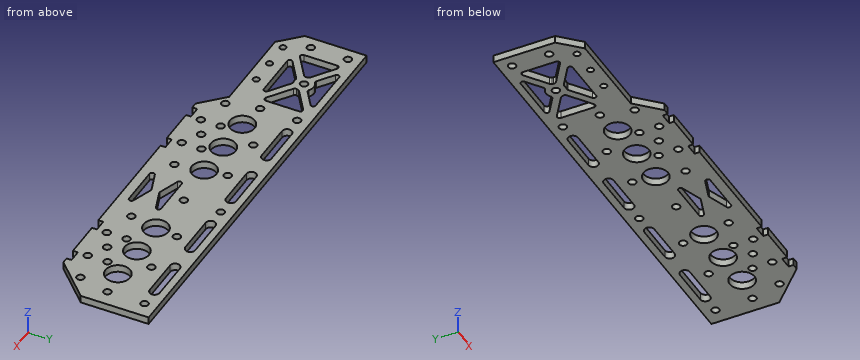
from build123d import *

# Parameters (mm, degrees)
SKETCH_1_R          = 1.55
SKETCH_1_R_2        = 1.3
EXTRUDE_1_DEPTH     = 3
FILLET_1_R          = 1
SKETCH_2_R          = 5
SKETCH_2_R_2        = 1.55
CUT_EXTRUDE_1_DEPTH = 10
SKETCH_3_W          = 5
SKETCH_3_H          = 8
CUT_EXTRUDE_2_DEPTH = 10


with BuildPart() as part:
    # 草图1 → 凸台-拉伸1 (new body)
    with BuildSketch(Plane.XY):
        Polygon((-68, 32), (103.45, 32), (103.45, 7), (103.45, 4.5), (88.907352941, -10), (86.4, -10), (-12.5, -10), (-15, -10), (-24.026470588, -1), (-60.023460411, -1), (-68, 7), align=None)
        with Locations((-7.5, 4)):
            Circle(SKETCH_1_R, mode=Mode.SUBTRACT)
        with Locations((-7.5, -4)):
            Circle(SKETCH_1_R, mode=Mode.SUBTRACT)
        with Locations((7.5, -4)):
            Circle(SKETCH_1_R, mode=Mode.SUBTRACT)
        with Locations((7.5, 4)):
            Circle(SKETCH_1_R, mode=Mode.SUBTRACT)
        with Locations((66.4, 4)):
            Circle(SKETCH_1_R, mode=Mode.SUBTRACT)
        with Locations((66.4, -4)):
            Circle(SKETCH_1_R, mode=Mode.SUBTRACT)
        with Locations((81.4, 4)):
            Circle(SKETCH_1_R, mode=Mode.SUBTRACT)
        with Locations((81.4, -4)):
            Circle(SKETCH_1_R, mode=Mode.SUBTRACT)
        with Locations((-63, 27)):
            Circle(SKETCH_1_R, mode=Mode.SUBTRACT)
        with Locations((-63, 12)):
            Circle(SKETCH_1_R, mode=Mode.SUBTRACT)
        with Locations((16.95, 19.5)):
            Circle(SKETCH_1_R, mode=Mode.SUBTRACT)
        with Locations((-3.05, 19.5)):
            Circle(SKETCH_1_R, mode=Mode.SUBTRACT)
        with Locations((-23.05, 27)):
            Circle(SKETCH_1_R, mode=Mode.SUBTRACT)
        with Locations((-23.05, 12)):
            Circle(SKETCH_1_R, mode=Mode.SUBTRACT)
        with Locations((36.95, 27)):
            Circle(SKETCH_1_R, mode=Mode.SUBTRACT)
        with Locations((36.95, 12)):
            Circle(SKETCH_1_R, mode=Mode.SUBTRACT)
        with Locations((56.95, 19.5)):
            Circle(SKETCH_1_R, mode=Mode.SUBTRACT)
        with Locations((76.95, 19.5)):
            Circle(SKETCH_1_R, mode=Mode.SUBTRACT)
        with Locations((96.95, 27)):
            Circle(SKETCH_1_R, mode=Mode.SUBTRACT)
        with Locations((96.95, 12)):
            Circle(SKETCH_1_R, mode=Mode.SUBTRACT)
        with Locations((-48, 3)):
            Circle(SKETCH_1_R_2, mode=Mode.SUBTRACT)
        with Locations((-37.5, 3)):
            Circle(SKETCH_1_R_2, mode=Mode.SUBTRACT)
        with Locations((-58.5, 3)):
            Circle(SKETCH_1_R_2, mode=Mode.SUBTRACT)
        with Locations((-43.05, 19.5)):
            Circle(SKETCH_1_R, mode=Mode.SUBTRACT)
        with Locations((93.9, -0.5)):
            Circle(SKETCH_1_R, mode=Mode.SUBTRACT)
        with Locations(Location((53.9, -0.5, 0), (0, 0, 180))):
            Circle(SKETCH_1_R, mode=Mode.SUBTRACT)
        with Locations(Location((-20, -0.5, 0), (0, 0, 180))):
            Circle(SKETCH_1_R, mode=Mode.SUBTRACT)
        with Locations((20, -0.5)):
            Circle(SKETCH_1_R, mode=Mode.SUBTRACT)
        with BuildLine():
            Line((-15.05, 29), (0.95, 29))
            ThreePointArc((0.95, 29), (2.95, 27), (0.95, 25))
            Line((0.95, 25), (-15.05, 25))
            ThreePointArc((-15.05, 25), (-17.05, 27), (-15.05, 29))
        make_face(mode=Mode.SUBTRACT)
        with BuildLine():
            Line((12.95, 29), (28.95, 29))
            ThreePointArc((28.95, 29), (30.95, 27), (28.95, 25))
            Line((28.95, 25), (12.95, 25))
            ThreePointArc((12.95, 25), (10.95, 27), (12.95, 29))
        make_face(mode=Mode.SUBTRACT)
        with BuildLine():
            Line((44.95, 29), (60.95, 29))
            ThreePointArc((60.95, 29), (62.95, 27), (60.95, 25))
            Line((60.95, 25), (44.95, 25))
            ThreePointArc((44.95, 25), (42.95, 27), (44.95, 29))
        make_face(mode=Mode.SUBTRACT)
        with BuildLine():
            Line((72.95, 29), (88.95, 29))
            ThreePointArc((88.95, 29), (90.95, 27), (88.95, 25))
            Line((88.95, 25), (72.95, 25))
            ThreePointArc((72.95, 25), (70.95, 27), (72.95, 29))
        make_face(mode=Mode.SUBTRACT)
        with BuildLine():
            Line((-30.662765464, 29), (-40.203557385, 22.310296148))
            ThreePointArc((-40.203557385, 22.310296148), (-43.03543461, 23.499973481), (-45.875900736, 22.330951259))
            Line((-45.875900736, 22.330951259), (-55.387234536, 29))
            Line((-55.387234536, 29), (-30.662765464, 29))
        make_face(mode=Mode.SUBTRACT)
        with BuildLine():
            Line((-55.387234536, 8), (-44.370821033, 15.724363392))
            ThreePointArc((-44.370821033, 15.724363392), (-43.032385745, 15.500038783), (-41.695978002, 15.736142347))
            Line((-41.695978002, 15.736142347), (-30.662765464, 8))
            Line((-30.662765464, 8), (-55.387234536, 8))
        make_face(mode=Mode.SUBTRACT)
        with BuildLine():
            Line((-58, 27.16801086), (-47.04998801, 19.490206126))
            ThreePointArc((-47.04998801, 19.490206126), (-46.950749965, 18.614477719), (-46.662143081, 17.781738565))
            Line((-46.662143081, 17.781738565), (-58, 9.83198914))
            Line((-58, 9.83198914), (-58, 27.16801086))
        make_face(mode=Mode.SUBTRACT)
        with BuildLine():
            Line((-39.425439217, 17.808090093), (-28.05, 9.83198914))
            Line((-28.05, 9.83198914), (-28.05, 27.16801086))
            Line((-28.05, 27.16801086), (-39.050253376, 19.454978443))
            ThreePointArc((-39.050253376, 19.454978443), (-39.149926133, 18.611504738), (-39.425439217, 17.808090093))
        make_face(mode=Mode.SUBTRACT)
        Polygon((23.014193592, -6), (36.95, -1.090366306), (50.885806408, -6), align=None, mode=Mode.SUBTRACT)
        Polygon((23.014193592, 7), (36.95, 2.090366306), (50.885806408, 7), align=None, mode=Mode.SUBTRACT)
    extrude(amount=EXTRUDE_1_DEPTH)

    # 圆角1
    fillet_1_edges = [part.edges().sort_by_distance(p)[0] for p in [
        (-30.662765464, 29, 1.5),
        (-55.387234536, 29, 1.5),
        (-45.875900736, 22.330951259, 1.5),
        (-40.203557385, 22.310296148, 1.5),
        (-55.387234536, 8, 1.5),
        (-30.662765464, 8, 1.5),
        (-41.695978002, 15.736142347, 1.5),
        (-44.370821033, 15.724363392, 1.5),
        (-58, 27.16801086, 1.5),
        (-58, 9.83198914, 1.5),
        (-46.662143081, 17.781738565, 1.5),
        (-47.04998801, 19.490206126, 1.5),
        (-28.05, 9.83198914, 1.5),
        (-28.05, 27.16801086, 1.5),
        (-39.050253376, 19.454978443, 1.5),
        (-39.425439217, 17.808090093, 1.5),
        (50.885806408, 7, 1.5),
        (23.014193592, 7, 1.5),
        (36.95, 2.090366306, 1.5),
        (23.014193592, -6, 1.5),
        (50.885806408, -6, 1.5),
        (36.95, -1.090366306, 1.5),
    ]]
    fillet(fillet_1_edges, radius=FILLET_1_R)

    # 草图2 → 切除-拉伸1 (cut)
    with BuildSketch(Plane.XY.offset(3)):
        with Locations((-12, 10.5)):
            Circle(SKETCH_2_R)
        with Locations((3, 10.5)):
            Circle(SKETCH_2_R)
        with Locations((18, 10.5)):
            Circle(SKETCH_2_R)
        with Locations(Location((55.907352941, 10.5, 0), (0, 0, 180))):
            Circle(SKETCH_2_R)
        with Locations(Location((70.907352941, 10.5, 0), (0, 0, 180))):
            Circle(SKETCH_2_R)
        with Locations(Location((85.907352941, 10.5, 0), (0, 0, 180))):
            Circle(SKETCH_2_R)
        Circle(SKETCH_2_R_2)
        with Locations(Location((73.907352941, 0, 0), (0, 0, 180))):
            Circle(SKETCH_2_R_2)
    extrude(amount=-CUT_EXTRUDE_1_DEPTH, mode=Mode.SUBTRACT)

    # 草图3 → 切除-拉伸2 (cut)
    with BuildSketch(Plane.XY.offset(3)):
        with Locations((-10, -12)):
            Rectangle(SKETCH_3_W, SKETCH_3_H)
        with Locations((10, -12)):
            Rectangle(SKETCH_3_W, SKETCH_3_H)
        with Locations((63.907352941, -12)):
            Rectangle(SKETCH_3_W, SKETCH_3_H)
        with Locations((83.907352941, -12)):
            Rectangle(SKETCH_3_W, SKETCH_3_H)
    extrude(amount=-CUT_EXTRUDE_2_DEPTH, mode=Mode.SUBTRACT)


solid = part.part
Geometry check sheet. Reference: the model listing, model coordinates, mm. Round coordinates to 2 decimals unless told otherwise and drop trailing zeros. Loops run counter-clockwise (first coordinate to the right, second up) from the corner with the lowest first, then second, coordinate; pieces in that order, holes last. Notation, with made-up numbers: (-21, 32) - (-7, 32) arc R14 ccw to (-7, 51) - close; hole circle Ø4 at (84, 7.25). An arc over 180 degrees is marked (long way). Answer as CSV lines item,"result".
(1) Cross-section at C-C, the plane z = 1.95. Give the number of separate pieces and of enclosed holes in the cut face, and give its area (3 significant figures).
Output values:
separate pieces,"1"
enclosed holes,"46"
area,"5,070 mm²"
(2) Depth check by flat-ended pin: pin 1 Ø3 at (x, y) = (-20, -0.5) entering from +Z. Enter the tip coordinate at first touch or a pass-through.
Output values:
pin 1,"passes through"
(3) Material ranges on line 1 along Y through (x, z) = (-43.05, 0.95); line 2 along Y through (x, z) = (96.95, 1.95); line 3 along Y through (x, z) = (15, 1.3), recorded low to high.
Output values:
line 1,"y = -1 to 8, 15.5 to 17.95, 21.05 to 23.5, 29 to 32"
line 2,"y = -1.98 to 10.45, 13.55 to 25.45, 28.55 to 32"
line 3,"y = -10 to 6.5, 14.5 to 25, 29 to 32"
(4) Cross-section at A-A, the plane x = 20. Enter the section's corners in (y, z).
Output values:
outline,"(-10, 0) - (-2.05, 0) - (-2.05, 3) - (-10, 3) - close; (1.05, 0) - (5.92, 0) - (5.92, 3) - (1.05, 3) - close; (15.08, 0) - (25, 0) - (25, 3) - (15.08, 3) - close; (29, 0) - (32, 0) - (32, 3) - (29, 3) - close"
